from build123d import *

# Parameters (mm, degrees)
SKETCH2_R           = 1.475
BOSS_EXTRUDE1_DEPTH = 0.254
FILLET1_R           = 6.35


with BuildPart() as part:
    # Sketch2 → Boss-Extrude1 (new body)
    # profile 1 of 3: a face of its own
    with BuildSketch(Plane.XY):
        with BuildLine():
            ThreePointArc((-6.35, -37.972720471), (-8.946176851, -37.446173633), (-11.5, -36.742346142))
            ThreePointArc((-11.5, -36.742346142), (-22.79802623, 31.024184115), (38.5, 0))
            ThreePointArc((38.5, 0), (31.024184115, -22.79802623), (11.5, -36.742346142))
            ThreePointArc((11.5, -36.742346142), (8.946176851, -37.446173633), (6.35, -37.972720471))
            Line((6.35, -37.972720471), (6.35, -47.5))
            Line((6.35, -47.5), (49.325, -47.5))
            Line((49.325, -47.5), (49.325, 47.5))
            Line((49.325, 47.5), (-49.325, 47.5))
            Line((-49.325, 47.5), (-49.325, -47.5))
            Line((-49.325, -47.5), (-6.35, -47.5))
            Line((-6.35, -47.5), (-6.35, -37.972720471))
        make_face()
        with Locations((-43, -43)):
            Circle(SKETCH2_R, mode=Mode.SUBTRACT)
        with Locations((43, -43)):
            Circle(SKETCH2_R, mode=Mode.SUBTRACT)
        with Locations((-43, 43)):
            Circle(SKETCH2_R, mode=Mode.SUBTRACT)
        with Locations((43, 43)):
            Circle(SKETCH2_R, mode=Mode.SUBTRACT)
    # profile 2 of 3: a face of its own
    with BuildSketch(Plane.XY):
        with BuildLine():
            Line((11.5, -36.742346142), (6.35, -36.742346142))
            Line((6.35, -36.742346142), (6.35, -37.972720471))
            ThreePointArc((6.35, -37.972720471), (8.946176851, -37.446173633), (11.5, -36.742346142))
        make_face()
    # profile 3 of 3: a face of its own
    with BuildSketch(Plane.XY):
        with BuildLine():
            Line((-6.35, -36.742346142), (-11.5, -36.742346142))
            ThreePointArc((-11.5, -36.742346142), (-8.946176851, -37.446173633), (-6.35, -37.972720471))
            Line((-6.35, -37.972720471), (-6.35, -36.742346142))
        make_face()
    extrude(amount=BOSS_EXTRUDE1_DEPTH)

    # Fillet1
    fillet1_edges = [part.edges().sort_by_distance(p)[0] for p in [
        (-49.325, -47.5, 0.127),
        (-49.325, 47.5, 0.127),
        (49.325, 47.5, 0.127),
        (49.325, -47.5, 0.127),
    ]]
    fillet(fillet1_edges, radius=FILLET1_R)


solid = part.part
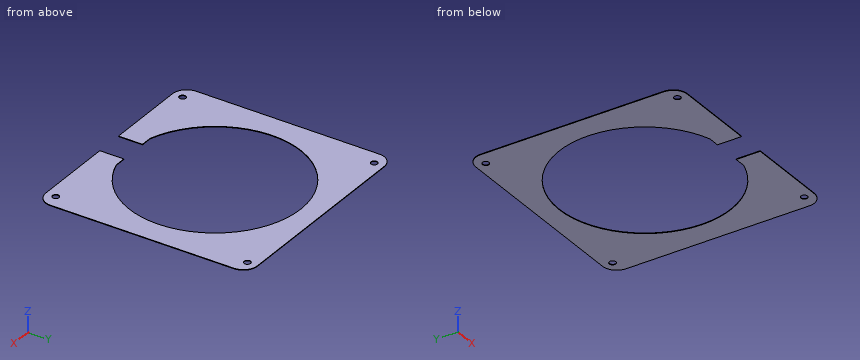
Design review of the part built by this model. Coordinates are the model's own, in mm. Coordinates: 2 decimals unless noted, no trailing zeros. Order: outer loops, then holes, each group sorted by start corner. A loop starts at its lowest first (then second) coordinate and runs counter-clockwise, first axis right, second up.
Item 1: Take a section at C-C, the plane y = -39. Write out the cut boundary in (x, z) (3 decimals).
Item 2: Take a section at A-A, the plane z = 0.2. Write out the cut boundary in (x, y) (3 decimals).
Item 3: For line 1 (Y direction, x = 43, z = 0.15) (3 decimals); line 2 (Y direction, x = -35.5, z = 0.2); line 3 (Y direction, x = -24, z = 0.2), list the stretches that pass through material, from the lowest coordinate up.
Item 4: Take a section at D-D, the plane y = 43. Write out the cut boundary in (x, z) (3 decimals), then the cut area to 3 significant figures.
Item 5: Take a section at B-B, the plane x = 29. Write out the cut boundary in (y, z), then the cut area to 3 significant figures.
The answers:
1. outline: (-49.325, 0) - (-6.35, 0) - (-6.35, 0.254) - (-49.325, 0.254) - close; (6.35, 0) - (49.325, 0) - (49.325, 0.254) - (6.35, 0.254) - close
2. outline: (-49.325, -41.15) arc R6.35 ccw to (-42.975, -47.5) - (-6.35, -47.5) - (-6.35, -36.742) - (-11.5, -36.742) arc R38.5 cw (long way) to (11.5, -36.742) - (6.35, -36.742) - (6.35, -47.5) - (42.975, -47.5) arc R6.35 ccw to (49.325, -41.15) - (49.325, 41.15) arc R6.35 ccw to (42.975, 47.5) - (-42.975, 47.5) arc R6.35 ccw to (-49.325, 41.15) - close; hole circle Ø2.95 at (-43, -43); hole circle Ø2.95 at (-43, 43); hole circle Ø2.95 at (43, -43); hole circle Ø2.95 at (43, 43)
3. line 1: y = -47.5 to -44.475, -41.525 to 41.525, 44.475 to 47.5
3. line 2: y = -47.5 to -14.9, 14.9 to 47.5
3. line 3: y = -47.5 to -30.1, 30.1 to 47.5
4. outline: (-49.05, 0) - (-44.475, 0) - (-44.475, 0.254) - (-49.05, 0.254) - close; (-41.525, 0) - (41.525, 0) - (41.525, 0.254) - (-41.525, 0.254) - close; (44.475, 0) - (49.05, 0) - (49.05, 0.254) - (44.475, 0.254) - close
4. area: 23.4 mm2
5. outline: (-47.5, 0) - (-25.32, 0) - (-25.32, 0.25) - (-47.5, 0.25) - close; (25.32, 0) - (47.5, 0) - (47.5, 0.25) - (25.32, 0.25) - close
5. area: 11.3 mm2
